Autodesk Inventor part; units mm, degrees
ref_plane "YZ Plane" through (0, 0, 0) normal (1, 0, 0) x (0, 1, 0)
ref_plane "XZ Plane" through (0, 0, 0) normal (0, 1, 0) x (-1, 0, 0)
ref_plane "XY Plane" through (0, 0, 0) normal (0, 0, 1) x (1, 0, 0)
sketch "Эскиз1" plane through (0, 0, 0) normal (0, 1, 0) x (-1, 0, 0)
  circle A0 centre (0, 0) radius 44
  circle A1 centre (0, 0) radius 4.25
  circle A2 centre (0, -38) radius 2.5
  circle A3 centre (38, 0) radius 2.5
  circle A4 centre (0, 38) radius 2.5
  circle A5 centre (-38, 0) radius 2.5
  dimension "d0" = 88
  dimension "d1" = 8.5
  dimension "d3" = 5
  dimension "d6" = 360
extrude "Выдавливание1" add sketch "Эскиз1" along normal blind 1
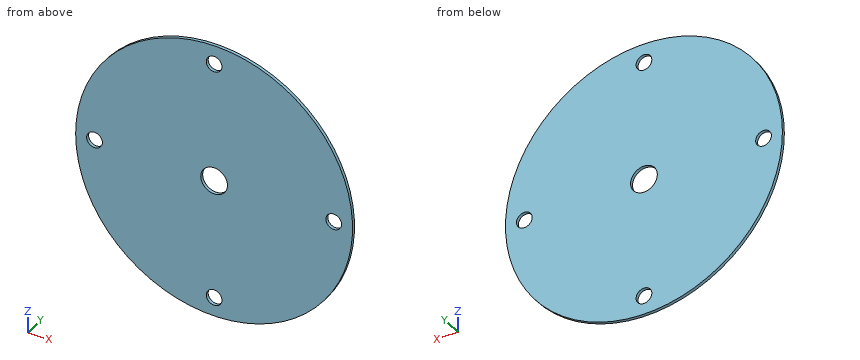
Can you work these out from the model? Positions are in its coordinate system, mm. Round coordinates to 2 decimals unless told otherwise and drop trailing zeros. Order: outer loops, then holes, each group sorted by start corner. A loop starts at its lowest first (then second) coordinate and runs counter-clockwise, first axis right, second up.
(1) If we section it at A-A (z = 0): Please give me the cut outline in (x, y).
Results are:
outline: (-44, 0) - (-40.5, 0) - (-40.5, 1) - (-44, 1) - close; (-35.5, 0) - (-4.25, 0) - (-4.25, 1) - (-35.5, 1) - close; (4.25, 0) - (35.5, 0) - (35.5, 1) - (4.25, 1) - close; (40.5, 0) - (44, 0) - (44, 1) - (40.5, 1) - close
(2) I'm going to push a flat-ended pin straight in: pin 1 (1.5 mm diameter, centred on x = -22.5, z = -22, fed in from -Y). Where does the tip first touch, or does it pass through?
Results are:
pin 1: stops at y = 0
(3) If we section it at D-D (z = -28.5): Please give me the cut outline in (x, y).
Results are:
outline: (-33.52, 0) - (33.52, 0) - (33.52, 1) - (-33.52, 1) - close
(4) If I drill on L1, parallel to Z at x = 0, y = 0.4; L2, parallel to X at y = 0.3, z = -1; L3, parallel to X at y = 0.3, z = -2, over which ranges is the centre line in solid material (lowest first)?
Results are:
L1: z = -44 to -40.5, -35.5 to -4.25, 4.25 to 35.5, 40.5 to 44
L2: x = -43.99 to -40.29, -35.71 to -4.13, 4.13 to 35.71, 40.29 to 43.99
L3: x = -43.95 to -39.5, -36.5 to -3.75, 3.75 to 36.5, 39.5 to 43.95
(5) If we section it at B-B (x = -37): Please give me the cut outline in (y, z).
Results are:
outline: (0, -23.81) - (1, -23.81) - (1, -2.29) - (0, -2.29) - close; (0, 2.29) - (1, 2.29) - (1, 23.81) - (0, 23.81) - close
(6) If we section it at C-C (z = -38): Please give me the cut outline in (x, y), plus the area to 3 significant figures.
Results are:
outline: (-22.18, 0) - (-2.5, 0) - (-2.5, 1) - (-22.18, 1) - close; (2.5, 0) - (22.18, 0) - (22.18, 1) - (2.5, 1) - close
area: 39.4 mm2
